```python
from build123d import *

# Parameters (mm, degrees)
SKIZZE2_W                       = 112.5
SKIZZE2_H                       = 109
AUFSATZ_LINEAR_AUSTRAGEN1_DEPTH = 2
SKIZZE3_W                       = 20.5
SKIZZE3_H                       = 20.5
SCHNITT_LINEAR_AUSTRAGEN1_DEPTH = 157.656471299
SKIZZE5_W                       = 91
SKIZZE5_H                       = 84.5
AUFSATZ_LINEAR_AUSTRAGEN2_DEPTH = 5
SKIZZE8_W                       = 21.5
SKIZZE8_H                       = 19
SCHNITT_LINEAR_AUSTRAGEN3_DEPTH = 157.723482606
SKIZZE9_W                       = 21.5
SKIZZE9_H                       = 69.5
AUFSATZ_LINEAR_AUSTRAGEN3_DEPTH = 5
FASE1_SIZE                      = 5
FASE1_SIZE2                     = 10.722534603
SKIZZE10_W                      = 85.75
SKIZZE10_H                      = 128
SCHNITT_LINEAR_AUSTRAGEN4_DEPTH = 3
VERRUNDUNG1_R                   = 1
DURCHGANGSLOCH_F_R_M41_D        = 4.5
DURCHGANGSLOCH_F_R_M41_DEPTH    = 6
VERRUNDUNG2_R                   = 1.5
SCHNITT_LINEAR_AUSTRAGEN7_DEPTH = 246.416482739


with BuildPart() as part:
    # Skizze2 → Aufsatz-Linear austragen1 (new body)
    with BuildSketch(Plane(origin=(0, 0, 0), x_dir=(1, 0, 0), z_dir=(0, 1, 0))):
        with Locations((-56.25, 54.5)):
            Rectangle(SKIZZE2_W, SKIZZE2_H)
    extrude(amount=AUFSATZ_LINEAR_AUSTRAGEN1_DEPTH)

    # Skizze3 → Schnitt-Linear austragen1 (cut, through all)
    with BuildSketch(Plane(origin=(0, 2, 0), x_dir=(1, 0, 0), z_dir=(0, 1, 0))):
        with Locations((-102.25, 98.75)):
            Rectangle(SKIZZE3_W, SKIZZE3_H)
    extrude(amount=-SCHNITT_LINEAR_AUSTRAGEN1_DEPTH, mode=Mode.SUBTRACT)

    # Skizze5 → Aufsatz-Linear austragen2 (add)
    with BuildSketch(Plane(origin=(0, 2, 0), x_dir=(1, 0, 0), z_dir=(0, 1, 0))):
        with Locations((-45.5, 42.25)):
            Rectangle(SKIZZE5_W, SKIZZE5_H)
    extrude(amount=AUFSATZ_LINEAR_AUSTRAGEN2_DEPTH)

    # Skizze8 → Schnitt-Linear austragen3 (cut, through all)
    with BuildSketch(Plane(origin=(0, 2, 0), x_dir=(1, 0, 0), z_dir=(0, 1, 0))):
        with Locations((-101.75, 79)):
            Rectangle(SKIZZE8_W, SKIZZE8_H)
    extrude(amount=-SCHNITT_LINEAR_AUSTRAGEN3_DEPTH, mode=Mode.SUBTRACT)

    # Skizze9 → Aufsatz-Linear austragen3 (add)
    with BuildSketch(Plane(origin=(0, 2, 0), x_dir=(1, 0, 0), z_dir=(0, 1, 0))):
        with Locations((-101.75, 34.75)):
            Rectangle(SKIZZE9_W, SKIZZE9_H)
    extrude(amount=AUFSATZ_LINEAR_AUSTRAGEN3_DEPTH)

    # Fase1
    fase1_edges = [part.edges().sort_by_distance(p)[0] for p in [
        (-91, 7, -77),
    ]]
    fase1_side = [part.faces().sort_by_distance(p)[0] for p in [
        (-91, 3.32300885, -77.672566372),
    ]]
    chamfer(fase1_edges, length=FASE1_SIZE, length2=FASE1_SIZE2, reference=fase1_side[0])

    # Skizze10 → Schnitt-Linear austragen4 (cut)
    with BuildSketch(Plane(origin=(0, 0, 0), x_dir=(1, 0, 0), z_dir=(0, 1, 0))):
        Rectangle(SKIZZE10_W, SKIZZE10_H)
    extrude(amount=SCHNITT_LINEAR_AUSTRAGEN4_DEPTH, mode=Mode.SUBTRACT)

    # Verrundung1
    verrundung1_edges = [part.edges().sort_by_distance(p)[0] for p in [
        (-42.875, 1.5, -64),
    ]]
    fillet(verrundung1_edges, radius=VERRUNDUNG1_R)

    # Durchgangsloch für M41
    with Locations(Plane(origin=(0, 0, 0), x_dir=(-1, 0, 0), z_dir=(0, -1, 0))):
        with Locations((67, 99)):
            Hole(DURCHGANGSLOCH_F_R_M41_D / 2, depth=DURCHGANGSLOCH_F_R_M41_DEPTH)

    # Verrundung2
    # the kernel refuses this fillet: 1.5 mm, written as the material it adds along each edge
    with BuildSketch(Plane(origin=(-91, 0, -69.5), x_dir=(-1, 0, 0), z_dir=(0, 1, 0))) as verrundung2_piece_1_section:
        with BuildLine():
            CenterArc((VERRUNDUNG2_R, -VERRUNDUNG2_R), VERRUNDUNG2_R, 90, 90)
            Line((0, -VERRUNDUNG2_R), (0, 0))
            Line((0, 0), (VERRUNDUNG2_R, 0))
        make_face()
    verrundung2_piece_1 = extrude(amount=5.75, mode=Mode.PRIVATE)
    verrundung2_piece_1 = split(verrundung2_piece_1, bisect_by=Plane(origin=(-91.766044443, 1.64278761, -69.5), z_dir=(0.4226182617406971, -0.906307787036651, 0)), keep=Keep.TOP, mode=Mode.PRIVATE)
    add(verrundung2_piece_1)
    # the kernel refuses this fillet: 1.5 mm, written as the material it takes off along each edge
    with BuildSketch(Plane(origin=(-92, 5.535533906, -88.5), x_dir=(0, 0, -1), z_dir=(0, -1, 0))) as verrundung2_2_piece_1:
        with BuildLine():
            CenterArc((1.414213562, 1.5), VERRUNDUNG2_R, 199.471220634, 70.528779366)
            Line((0, 1), (0, 0))
            Line((0, 0), (1.414213562, 0))
        make_face()
    extrude(amount=9.071067812, mode=Mode.SUBTRACT)
    with BuildSketch(Plane(origin=(-112.5, 10.75, -69.5), x_dir=(1, 0, 0), z_dir=(0, -1, 0))) as verrundung2_2_piece_2:
        with BuildLine():
            CenterArc((VERRUNDUNG2_R, VERRUNDUNG2_R), VERRUNDUNG2_R, 180, 90)
            Line((0, VERRUNDUNG2_R), (0, 0))
            Line((0, 0), (VERRUNDUNG2_R, 0))
        make_face()
    extrude(amount=14.5, mode=Mode.SUBTRACT)
    with BuildSketch(Plane(origin=(-92, 5.75, -109), x_dir=(1, 0, 0), z_dir=(0, -1, 0))) as verrundung2_2_piece_3:
        with BuildLine():
            CenterArc((VERRUNDUNG2_R, VERRUNDUNG2_R), VERRUNDUNG2_R, 180, 90)
            Line((0, VERRUNDUNG2_R), (0, 0))
            Line((0, 0), (VERRUNDUNG2_R, 0))
        make_face()
    extrude(amount=9.5, mode=Mode.SUBTRACT)

    # Spiegeln1: part across face


with BuildPart() as part_1:
    add(part.part)
    add(part.part.mirror(Plane(origin=(-63.046065737, 3.890438247, 0), x_dir=(1, 0, 0), z_dir=(0, 0, 1))))

    # Spiegeln2: part across plane


with BuildPart() as part_2:
    add(part_1.part)
    add(part_1.part.mirror(Plane(origin=(0, 2, 0), x_dir=(0, 0, 1), z_dir=(-1, 0, 0))))

    # Skizze15 → Schnitt-Linear austragen7 (cut, through all)
    with BuildSketch(Plane(origin=(0, 0, -109), x_dir=(-1, 0, 0), z_dir=(0, 0, -1))):
        Polygon((0, 0), (4.171137574, 3.5), (0, 7), (-112.5, 7), (-112.5, 0), align=None)
    extrude(amount=-SCHNITT_LINEAR_AUSTRAGEN7_DEPTH, mode=Mode.SUBTRACT)


solid = part_2.part
```
Design review of the part built by this model. Coordinates are the model's own, in mm. A direction names the side the tool comes from. Coordinates: 2 decimals unless noted, no trailing zeros. Order: outer loops, then holes, each group sorted by start corner. A loop starts at its lowest first (then second) coordinate and runs counter-clockwise, first axis right, second up.
1) Take a section at D-D, the plane z = 21.5. Give the boundary of the cut face in (x, y) (3 decimals), and give its area (3 significant figures).
2) Take a section at B-B, the plane x = -67. Give the boundary of the cut face in (y, z).
3) Clearance check with flat-ended pins moving along their axes: pin 1 (1 mm diameter, centred on y = 1.5, z = -75.5, fed in from -X); pin 2 (2 mm diameter, centred on y = 3.5, z = 78.5, fed in from +X); pin 3 (2 mm diameter, centred on y = 1, z = -99, fed in from -X). State where each tip first meets the part, or that it passes through.
4) Mouldability with a two-part tool opening along X and no side actions: class faces 4 (the cylindrical face through (-67.488, 1.014, -96.804)), 5 (the flat face through (-55, 0, -2)), 6 (the flat face through (-2.11, 5.23, -1.18)) as +X half, -X half, draft (parallel to the pull), parting line (faces both ways), or undercut.
5) Take a section at A-A, the plane z = -99. Give the boundary of the cut face in (x, y).
6) Take a section at C-C, the plane x = -55.5. Give the boundary of the cut face in (y, z), and give its area (3 significant figures).
7) For faces 1 (the flat face through (-23, 3, 1)), 2 (the flat face through (-47, 2, 97)), 3 (the flat face through (-45, 4, -84.5)), list the 3-axis set-ups (+Z, -Z, +X, -X, +Y, -Y) from which the entire face can be reached by the end or side of a thin tool; tool diameter is ignored.
8) Wall thickness on line 1 along Z through (x, y) = (-67, 0.45); line 2 along Z through (x, y) = (-33, 1.25); line 3 along X through (y, z) = (0.5, 10) (3 decimals): over which ranges is each line inside the solid? List them lowest first.
Returned:
1. outline: (-112.5, 0) - (-42.875, 0) - (-42.875, 3) - (-3.575, 3) - (-4.171, 3.5) - (0, 7) - (-112.5, 7) - close
1. area: 650 mm2
2. outline: (0, -109) - (2, -109) - (2, -101.25) - (0, -101.25) - close; (0, -96.75) - (2, -96.75) - (2, -84.5) - (7, -84.5) - (7, 84.5) - (2, 84.5) - (2, 96.75) - (0, 96.75) - close; (0, 101.25) - (2, 101.25) - (2, 109) - (0, 109) - close
3. pin 1: stops at x = -91
3. pin 2: stops at x = -2.98
3. pin 3: stops at x = -92
4. face 4: undercut
4. face 5: draft
4. face 6: +X half
5. outline: (-92, 0) - (-69.25, 0) - (-69.25, 2) - (-92, 2) - close; (-64.75, 0) - (0, 0) - (-2.38, 2) - (-64.75, 2) - close
6. outline: (0, -109) - (2, -109) - (2, -84.5) - (7, -84.5) - (7, 84.5) - (2, 84.5) - (2, 109) - (0, 109) - close
6. area: 1,280 mm2
7. face 1: +X, -Y
7. face 2: +Z, +X, -X, +Y
7. face 3: -Z, +X, -X, +Y
8. line 1: z = -109 to -101.25, -96.75 to 96.75, 101.25 to 109
8. line 2: z = -109 to -64, 64 to 109
8. line 3: x = -112.5 to -42.875
